from build123d import *

# Parameters (mm, degrees)
F0_W     = 127
F0_H     = 25.4
F1_DEPTH = 25.4
F2_W     = 17.595317
F2_H     = 25.4
F3_DEPTH = 25.4
F4_W     = 17.595317
F4_H     = 6.35
F5_DEPTH = 19.05
F6_R     = 5.08
F7_R     = 5.08


with BuildPart() as f1:
    # F0 (on Front) → F1 (new body)
    with BuildSketch(Plane.XZ):
        with Locations((63.5, 12.7)):
            Rectangle(F0_W, F0_H)
    extrude(amount=-F1_DEPTH)

    # F2 (on face) → F3 (join)
    with BuildSketch(Plane.XZ):
        with Locations((8.797658, 12.7)):
            Rectangle(F2_W, F2_H)
    extrude(amount=F3_DEPTH)

    # F4 (on face) → F5 (cut)
    with BuildSketch(Plane.XZ.offset(25.4)):
        with Locations((8.797658, 12.076512)):
            Rectangle(F4_W, F4_H)
    extrude(amount=-F5_DEPTH, mode=Mode.SUBTRACT)

    # F6
    f6_edges = [f1.edges().sort_by_distance(p)[0] for p in [
        (8.797659, -25.4, 25.4),
        (8.797659, -25.4, 0),
        (127, 0, 12.7),
        (127, 25.4, 12.7),
    ]]
    fillet(f6_edges, radius=F6_R)

    # F7
    f7_edges = [f1.edges().sort_by_distance(p)[0] for p in [
        (0, 25.4, 12.7),
    ]]
    fillet(f7_edges, radius=F7_R)


solid = f1.part
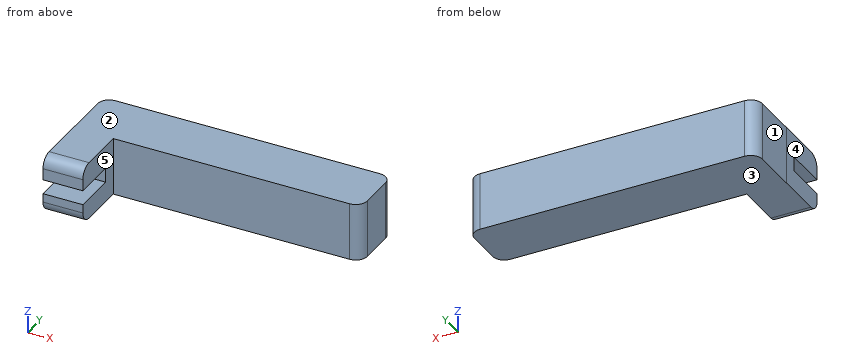
For this review, take the finished solid that the model builds, in its own axes (mm). Face numbers are marked on the shaded views. A direction names the side the tool comes from. Round coordinates to 2 decimals unless told otherwise and drop trailing zeros. Write each loop counter-clockwise with the first axis right and the second up, starting at its lowest first coordinate (ties: lowest second). Pieces come first, ordered by that corner, then holes. Notation, with made-up numbers: (2, -28) -> (20, -28) arc R22 ccw to (20, 2) -> close; hole circle Ø10 at (32, -24.5). An arc over 180 degrees is marked (long way). Put each result on its own line as item: value.
Q1. To check wall thickness, follow L1, parallel to Y at x = 87, z = 8.75; L2, parallel to X at y = -17, z = 3; L3, parallel to X at y = 1, z = 22.5. State the ranges of each line that lie inside material, in increasing order. Write a range as [from, to].
Determined:
L1: y = [0, 25.4]
L2: x = [0, 17.6]
L3: x = [0, 124.95]
Q2. Clearance check with flat-ended pins moving along their axes: pin 1 Ø1 at (y, z) = (4.5, 8) entering from +X; pin 2 Ø1 at (x, z) = (14.5, 14) entering from -Y; pin 3 Ø2 at (x, z) = (39, 18) entering from -Y. State where each tip first meets the part, or that it passes through.
Determined:
pin 1: stops at x = 127
pin 2: stops at y = -6.35
pin 3: stops at y = 0
Q3. Consider section A-A on y = -18. State the section outline as (x, z) points, and give its area (3 significant figures).
Determined:
outline: (0, 0) -> (17.6, 0) -> (17.6, 8.9) -> (0, 8.9) -> close; (0, 15.25) -> (17.6, 15.25) -> (17.6, 25.4) -> (0, 25.4) -> close
area: 335 mm^2
Q4. The part is to be moulded in two halves that separate along Z. For the marked faces 1, 2 and 3, say which applies: released by +Z, released by -Z, zero draft, split by the parting line, or undercut.
Determined:
face 1: zero draft
face 2: released by +Z
face 3: released by -Z
Q5. Machinability: for the marked faces 4 and 5, which of the approach directions +Z, -Z, +X, -X, +Y, -Y give a long, thin tool a straight path to every point of the face, cutting with its end or side? Answer none if there is none.
Determined:
face 4: +Z, -Z, -X, +Y, -Y
face 5: +Z, -Z, +X, -Y
Q6. Consider section B-B on z = 12.5. State the section outline as (x, y) points, and give its area (3 significant figures).
Determined:
outline: (0, -6.35) -> (17.6, -6.35) -> (17.6, 0) -> (121.92, 0) arc R5.08 ccw to (127, 5.08) -> (127, 20.32) arc R5.08 ccw to (121.92, 25.4) -> (5.08, 25.4) arc R5.08 ccw to (0, 20.32) -> close
area: 3,320 mm^2
Q7. Consider section C-C on x = 45. State the section outline as (y, z) points, and give its area (3 significant figures).
Determined:
outline: (0, 0) -> (25.4, 0) -> (25.4, 25.4) -> (0, 25.4) -> close
area: 645 mm^2
